Drawing for the job (mm, zero at the part's lowest x, y, z). Round coordinates to 2 decimals unless told otherwise and drop trailing zeros. Write each loop counter-clockwise with the first axis right and the second up, starting at its lowest first coordinate (ties: lowest second). Pieces come first, ordered by that corner, then holes. Notation, with made-up numbers: (-10, -5) - (4, -5) arc R31 ccw to (4, 33) - close; hole circle Ø6 at (22, 44.5). An arc over 180 degrees is marked (long way). Answer in a Markdown table with one row per item.
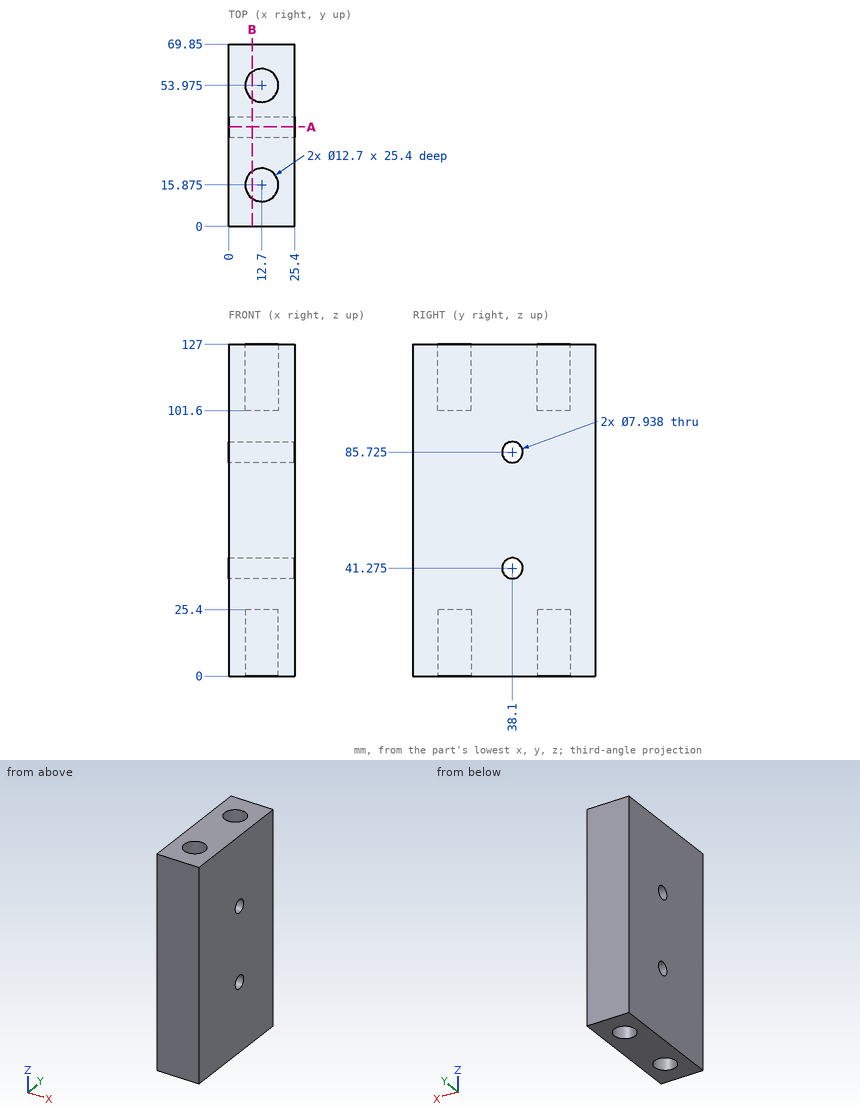
Q1. Drill centre lines: line 1 (Z direction, x = 14.5, y = 41) (1 decimal); line 2 (X direction, y = 16, z = 12); line 3 (Z direction, x = 12.5, y = 54). Where is each one in solid material? Low to high.
Computed:
| item | result |
|---|---|
| line 1 | z = 0 to 38.6, 44 to 83, 88.4 to 127 |
| line 2 | x = 0 to 6.35, 19.05 to 25.4 |
| line 3 | z = 25.4 to 101.6 |
Q2. Saw through at B-B on x = 9. Count the separate pieces of the cut face and the enclosed holes in it, then the cut area to 3 significant figures.
Computed:
| item | result |
|---|---|
| separate pieces | 1 |
| enclosed holes | 2 |
| area | 7,720 mm2 |
Q3. Flat gauge pins, fed straight in: pin 1 (4 mm diameter, centred on x = 11, y = 16, fed in from +Z); pin 2 (10 mm diameter, centred on x = 13, y = 17, fed in from -Z). Where does each tip first touch, or does it go through?
Computed:
| item | result |
|---|---|
| pin 1 | stops at z = 101.6 |
| pin 2 | stops at z = 25.4 |
Q4. Saw through at A-A on y = 38.1. List the corners of the cut face in (x, z).
Computed:
| item | result |
|---|---|
| outline | (0, 0) - (25.4, 0) - (25.4, 37.31) - (0, 37.31) - close; (0, 45.24) - (25.4, 45.24) - (25.4, 81.76) - (0, 81.76) - close; (0, 89.69) - (25.4, 89.69) - (25.4, 127) - (0, 127) - close |
